```python
from build123d import *

# Parameters (mm, degrees)
F0_W          = 3.56
F0_H          = 0.15
F1_DEPTH      = 1.98
F1_DEPTH_BACK = 1.98
F3_DEPTH      = 25
F4_W          = 1.269972
F4_H          = 0.792
F5_DEPTH      = 25


with BuildPart() as f1:
    # F0 (on Front) → F1 (new body, two sides)
    with BuildSketch(Plane.XZ) as f1_sk:
        with Locations((0, 0.075)):
            Rectangle(F0_W, F0_H)
        Polygon((-4.78, 0.923934), (-1.78, 0), (-1.78, 0.15), (-4.673934, 1.03), align=None)
        Polygon((1.78, 0.15), (1.78, 0), (4.78, 0.923934), (4.673934, 1.03), align=None)
    extrude(amount=F1_DEPTH)
    extrude(f1_sk.sketch, amount=-F1_DEPTH_BACK)

    # F2 (on face) → F3 (cut)
    with BuildSketch(Plane.XY.offset(0.15)):
        with BuildLine():
            ThreePointArc((-4.78, 1.188), (-4.548029, 1.748029), (-3.988, 1.98))
            Line((-3.988, 1.98), (-3.981051, 2.372488))
            Line((-3.981051, 2.372488), (-5.453913, 2.372488))
            Line((-5.453913, 2.372488), (-5.453913, -2.307775))
            Line((-5.453913, -2.307775), (-3.988, -2.307775))
            Line((-3.988, -2.307775), (-3.988, -1.98))
            ThreePointArc((-3.988, -1.98), (-4.548029, -1.748029), (-4.78, -1.188))
            ThreePointArc((-4.78, -1.188), (-4.548029, -0.627972), (-3.988, -0.396))
            Line((-3.988, -0.396), (-1.78, -0.396))
            Line((-1.78, -0.396), (-1.78, 0))
            Line((-1.78, 0), (-1.78, 0.396))
            Line((-1.78, 0.396), (-3.988, 0.396))
            ThreePointArc((-3.988, 0.396), (-4.548029, 0.627972), (-4.78, 1.188))
        make_face()
        with BuildLine():
            ThreePointArc((3.988, -0.396), (4.548029, -0.627972), (4.78, -1.188))
            ThreePointArc((4.78, -1.188), (4.548029, -1.748029), (3.988, -1.98))
            Line((3.988, -1.98), (3.988, -2.307775))
            Line((3.988, -2.307775), (5.453913, -2.307775))
            Line((5.453913, -2.307775), (5.453913, 2.372488))
            Line((5.453913, 2.372488), (3.981051, 2.372488))
            Line((3.981051, 2.372488), (3.988, 1.98))
            ThreePointArc((3.988, 1.98), (4.548029, 1.748029), (4.78, 1.188))
            ThreePointArc((4.78, 1.188), (4.548029, 0.627972), (3.988, 0.396))
            Line((3.988, 0.396), (1.78, 0.396))
            Line((1.78, 0.396), (1.78, 0))
            Line((1.78, 0), (1.78, -0.396))
            Line((1.78, -0.396), (3.988, -0.396))
        make_face()
    extrude(amount=F3_DEPTH, mode=Mode.SUBTRACT)

    # F4 (on face) → F5 (cut)
    with BuildSketch(Plane.XY.offset(0.15)):
        with Locations((-2.414986, 0)):
            Rectangle(F4_W, F4_H)
        with Locations((2.414986, 0)):
            Rectangle(F4_W, F4_H)
    extrude(amount=-F5_DEPTH, mode=Mode.SUBTRACT)


solid = f1.part
```
Work out the finished part from the listing and answer in its coordinate system (mm). Give positions to 0.01 mm unless a question says otherwise; leave off trailing zeros. Write each loop counter-clockwise with the first axis right and the second up, starting at its lowest first coordinate (ties: lowest second). Pieces come first, ordered by that corner, then holes.
(1) The part is cut by section D-D on x = 1.5. Write down the section's boundary in (y, z), plus the area to 3 significant figures.
Final values:
outline: (-1.98, 0) - (1.98, 0) - (1.98, 0.15) - (-1.98, 0.15) - close
area: 0.594 mm2
(2) The part is cut by section B-B on x = 3.25. Write down the section's boundary in (y, z).
Final values:
outline: (-1.98, 0.45) - (-0.4, 0.45) - (-0.4, 0.6) - (-1.98, 0.6) - close; (0.4, 0.45) - (1.98, 0.45) - (1.98, 0.6) - (0.4, 0.6) - close
(3) A flat-ended cylindrical pin translates along its axis: pin 1 Ø2 at (x, y) = (1, -1.5) entering from -Z. Find the tip coordinate at first contact, or state that the pin passes through.
Final values:
pin 1: stops at z = 0
(4) Straight lines are drawn through the part: line 1 (Z direction, x = -0.5, y = 0.3); line 2 (Y direction, x = 4.25, z = 0.85). For each, find the intervals that lie inside material, in ascending order.
Final values:
line 1: z = 0 to 0.15
line 2: y = -1.94 to -0.44, 0.44 to 1.94
(5) The part is cut by section A-A on z = 0.45. Write down the section's boundary in (x, y).
Final values:
outline: (-3.24, -1.98) - (-2.77, -1.98) - (-2.77, -0.4) - (-3.24, -0.4) - close; (-3.24, 0.4) - (-2.77, 0.4) - (-2.77, 1.98) - (-3.24, 1.98) - close; (2.77, -1.98) - (3.24, -1.98) - (3.24, -0.4) - (2.77, -0.4) - close; (2.77, 0.4) - (3.24, 0.4) - (3.24, 1.98) - (2.77, 1.98) - close
(6) The part is cut by section C-C on y = 1.45. Write down the section's boundary in (x, z).
Final values:
outline: (-4.74, 0.91) - (-1.78, 0) - (1.78, 0) - (4.74, 0.91) - (4.74, 0.97) - (4.67, 1.03) - (1.78, 0.15) - (-1.78, 0.15) - (-4.67, 1.03) - (-4.74, 0.97) - close
